Here's how the part is built. I have some questions about the finished solid (model axes, mm). Face numbers are marked on the shaded views. Round coordinates to 2 decimals unless told otherwise and drop trailing zeros. Loops run counter-clockwise (first coordinate to the right, second up) from the corner with the lowest first, then second, coordinate; pieces in that order, holes last. Notation, with made-up numbers: M 18.5,-28 L 59.5,-28 A14 cw 59.5,-23 Z; hole C 75,40 d5. An arc over 180 degrees is marked long. One line per question, with ' | ' between items. Start each with the question number.
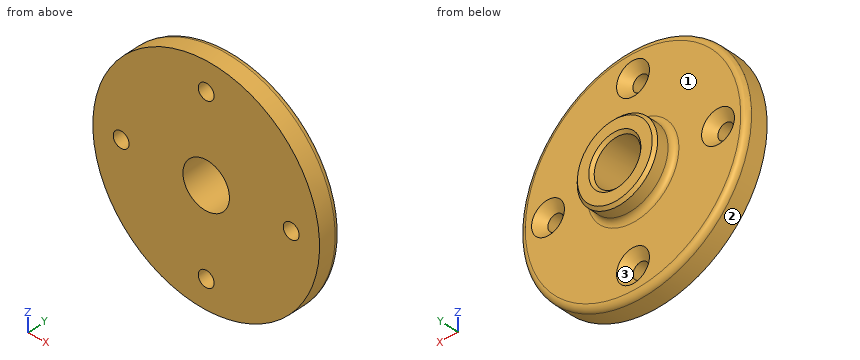
```python
from build123d import *

# Parameters (mm, degrees)
SKETCH1_R                    = 20
BOSS_EXTRUDE1_DEPTH          = 4
SKETCH2_R                    = 4.1
CUT_EXTRUDE1_DEPTH           = 29.565713714
SKETCH3_R                    = 1.4
CUT_EXTRUDE2_DEPTH           = 29.565713714
CHAMFER1_SIZE                = 1.5
CIRPATTERN1_COUNT            = 4
CHAMFER1_OF_CIRPATTERN1_SIZE = 1.5
FILLET1_R                    = 1
BOSS_EXTRUDE2_START          = 3.5
SKETCH4_R                    = 7.1
SKETCH4_R_2                  = 4.1
BOSS_EXTRUDE2_DEPTH          = 3.5
CHAMFER2_SIZE                = 0.5
FILLET2_R                    = 1
CHAMFER3_SIZE                = 0.5


with BuildPart() as part:
    # Sketch1 → Boss-Extrude1 (new body)
    with BuildSketch(Plane(origin=(0, 0, 0), x_dir=(1, 0, 0), z_dir=(0, 1, 0))):
        with Locations(Location((0, 0, 0), (0, 0, 270))):
            Circle(SKETCH1_R)
    extrude(amount=BOSS_EXTRUDE1_DEPTH)

    # Sketch2 → Cut-Extrude1 (cut, through all)
    with BuildSketch(Plane(origin=(0, 4, 0), x_dir=(1, 0, 0), z_dir=(0, 1, 0))):
        with Locations(Location((0, 0, 0), (0, 0, 270))):
            Circle(SKETCH2_R)
    extrude(amount=-CUT_EXTRUDE1_DEPTH, mode=Mode.SUBTRACT)

    # Sketch3 → Cut-Extrude2 (cut, through all)
    with BuildSketch(Plane(origin=(0, 4, 0), x_dir=(1, 0, 0), z_dir=(0, 1, 0))):
        with Locations(Location((0, 15, 0), (0, 0, 270))):
            Circle(SKETCH3_R)
    cut_extrude2 = extrude(amount=-CUT_EXTRUDE2_DEPTH, mode=Mode.SUBTRACT)

    # Chamfer1
    chamfer1_edges = [part.edges().sort_by_distance(p)[0] for p in [
        (0, 4, -16.4),
    ]]
    chamfer(chamfer1_edges, length=CHAMFER1_SIZE)

    # CirPattern1: Cut-Extrude2 ×4 about axis
    cirpattern1_axis = Axis((0, 0, 0), (0, 1, 0))
    for i in range(1, CIRPATTERN1_COUNT):
        add(cut_extrude2.rotate(cirpattern1_axis, i * 360 / CIRPATTERN1_COUNT), mode=Mode.SUBTRACT)

    # Chamfer1 of CirPattern1
    chamfer1_of_cirpattern1_edges = [part.edges().sort_by_distance(p)[0] for p in [
        (-16.4, 4, 0),
        (0, 4, 16.4),
        (16.4, 4, 0),
    ]]
    chamfer(chamfer1_of_cirpattern1_edges, length=CHAMFER1_OF_CIRPATTERN1_SIZE)

    # Fillet1
    fillet1_edges = [part.edges().sort_by_distance(p)[0] for p in [
        (0, 4, -20),
    ]]
    fillet(fillet1_edges, radius=FILLET1_R)

    # Sketch4 → Boss-Extrude2 (add)
    with BuildSketch(Plane(origin=(0, 4, 0), x_dir=(1, 0, 0), z_dir=(0, 1, 0)).offset(BOSS_EXTRUDE2_START)):
        with Locations(Location((0, 0, 0), (0, 0, 270))):
            Circle(SKETCH4_R)
        with Locations(Location((0, 0, 0), (0, 0, 270))):
            Circle(SKETCH4_R_2, mode=Mode.SUBTRACT)
    extrude(amount=-BOSS_EXTRUDE2_DEPTH)

    # Chamfer2
    chamfer2_edges = [part.edges().sort_by_distance(p)[0] for p in [
        (0, 7.5, -4.1),
    ]]
    chamfer(chamfer2_edges, length=CHAMFER2_SIZE)

    # Fillet2
    fillet2_edges = [part.edges().sort_by_distance(p)[0] for p in [
        (0, 4, -7.1),
    ]]
    fillet(fillet2_edges, radius=FILLET2_R)

    # Chamfer3
    chamfer3_edges = [part.edges().sort_by_distance(p)[0] for p in [
        (0, 7.5, -7.1),
    ]]
    chamfer(chamfer3_edges, length=CHAMFER3_SIZE)


solid = part.part
```
1) I'm going to push flat-ended pins straight in: pin 1 Ø3 at (x, z) = (-5, 12) entering from +Y; pin 2 Ø3.5 at (x, z) = (-15, 0) entering from +Y. Where does each tip first touch, or does it pass through?
2) We'd pull the mould along X, two halves only. Please class the marked faces 1, 2 and 3: pulls with the +X half, pulls with the -X half, needs draft (parallel to the pull), parting line crosses it, or undercut.
3) Imagine slicing it at A-A (z = 0). State how many separate pieces and enclosed holes the cut face has, then the cut area to 3 significant figures.
4) Imagine slicing it at C-C (y = 4.5). Write out the boundary of the cut face in (x, z), then the cut area to 3 significant figures.
5) Please list where these lines run through material, in increasing order: L1, parallel to Y at x = 3, z = -9.5; L2, parallel to Z at x = -15, y = 2.75; L3, parallel to X at y = 0.8, z = -15. Write a range as from..to.
Results are:
1) pin 1: y = 4 | pin 2: y = 2.85
2) face 1: needs draft | face 2: parting line crosses it | face 3: undercut
3) separate pieces: 4 | enclosed holes: 0 | area: 121 mm²
4) outline: C 0,0 d14.47; hole C 0,0 d8.2 | area: 112 mm²
5) L1: 0..4 | L2: -13.23..-1.65, 1.65..13.23 | L3: -13.23..-1.4, 1.4..13.23
